Source: CAD feature listing. Evaluate the final solid. Frame: model axes, mm. A direction names the side the tool comes from. Give positions to 0.01 mm unless a question says otherwise; leave off trailing zeros. Loops run counter-clockwise (first coordinate to the right, second up) from the corner with the lowest first, then second, coordinate; pieces in that order, holes last.
from build123d import *

# Parameters (mm, degrees)
SKETCH1_W               = 120
SKETCH1_H               = 100
BOSS_EXTRUDE1_DEPTH     = 5
SKETCH2_R               = 2.5
CUT_EXTRUDE1_DEPTH      = 6
CUT_EXTRUDE3_DEPTH      = 10
BOSS_EXTRUDE3_DEPTH     = 29.25
SKETCH8_W               = 20
SKETCH8_H               = 5
BOSS_EXTRUDE4_DEPTH     = 34.25
BOSS_EXTRUDE5_DEPTH     = 5
SKETCH11_W              = 5
SKETCH11_H              = 73
CUT_EXTRUDE6_DEPTH      = 1
CUT_EXTRUDE6_DEPTH_BACK = 120.837603572
SKETCH12_R              = 1.5
CUT_EXTRUDE7_DEPTH      = 69
CUT_EXTRUDE7_DEPTH_BACK = 6
SKETCH13_W              = 71.438611392
SKETCH13_H              = 5
BOSS_EXTRUDE6_DEPTH     = 10
SKETCH14_R              = 1.5
CUT_EXTRUDE8_DEPTH      = 30.25
SKETCH15_W              = 5
SKETCH15_H              = 14.999673458
SKETCH15_H_2            = 15
BOSS_EXTRUDE7_DEPTH     = 10
SKETCH17_R              = 1.5
CUT_EXTRUDE9_DEPTH      = 30.25


with BuildPart() as part:
    # Sketch1 → Boss-Extrude1 (new body)
    with BuildSketch(Plane.XY):
        with Locations((60, 50)):
            Rectangle(SKETCH1_W, SKETCH1_H)
    extrude(amount=BOSS_EXTRUDE1_DEPTH)

    # Sketch2 → Cut-Extrude1 (cut, through all)
    with BuildSketch(Plane.XY.offset(5)):
        with Locations((48.561388608, 53.909722104)):
            Circle(SKETCH2_R)
        with BuildLine():
            ThreePointArc((83.119368898, 4.555811435), (92.903152754, 13.119153924), (100.621925378, 23.582127225))
            ThreePointArc((100.621925378, 23.582127225), (96.02283809, 41.016960064), (78.588005251, 36.417872775))
            ThreePointArc((78.588005251, 36.417872775), (74.136099049, 30.383211826), (68.493169771, 25.444188565))
            ThreePointArc((68.493169771, 25.444188565), (65.36208077, 7.686900437), (83.119368898, 4.555811435))
        make_face()
    extrude(amount=-CUT_EXTRUDE1_DEPTH, mode=Mode.SUBTRACT)

    # Sketch5 → Cut-Extrude3 (cut)
    with BuildSketch(Plane.XY.offset(5)):
        with BuildLine():
            Line((120, 73), (48.561388608, 73))
            ThreePointArc((48.561388608, 73), (36.862057433, 68.994958603), (30.071644393, 58.660308282))
            Line((30.071644393, 58.660308282), (15, 0))
            Line((15, 0), (0, 0))
            Line((0, 0), (0, 100))
            Line((0, 100), (120, 100))
            Line((120, 100), (120, 73))
        make_face()
    extrude(amount=-CUT_EXTRUDE3_DEPTH, mode=Mode.SUBTRACT)

    # Sketch7 → Boss-Extrude3 (add)
    with BuildSketch(Plane(origin=(0, 0, 0), x_dir=(-1, 0, 0), z_dir=(0, 0, -1))):
        Polygon((-15, 0), (-30.123935814, 58.863831587), (-34.614250087, 56.248022366), (-20.162396428, 0), align=None)
        with BuildLine():
            Line((-120, 73), (-48.561388608, 73))
            ThreePointArc((-48.561388608, 73), (-45.276527497, 72.715263777), (-42.089655421, 71.869548932))
            Line((-42.089655421, 71.869548932), (-44.799142753, 68))
            Line((-44.799142753, 68), (-120, 68))
            Line((-120, 68), (-120, 73))
        make_face()
    extrude(amount=BOSS_EXTRUDE3_DEPTH)

    # Sketch8 → Boss-Extrude4 (add, through all)
    with BuildSketch(Plane(origin=(0, 0, -29.25), x_dir=(-1, 0, 0), z_dir=(0, 0, -1))):
        with Locations((-10.162396428, 2.5)):
            Rectangle(SKETCH8_W, SKETCH8_H)
    extrude(amount=-BOSS_EXTRUDE4_DEPTH)

    # Sketch10 → Boss-Extrude5 (add)
    with BuildSketch(Plane(origin=(0, 0, 0), x_dir=(-1, 0, 0), z_dir=(0, 0, -1))):
        with BuildLine():
            Line((-45.069655622, 67.613667586), (-42.089655421, 71.869548932))
            ThreePointArc((-42.089655421, 71.869548932), (-34.697505551, 66.663289264), (-30.124971237, 58.863228407))
            Line((-30.124971237, 58.863228407), (-34.614250087, 56.248022366))
            ThreePointArc((-34.614250087, 56.248022366), (-38.409874026, 63.248233001), (-45.069655622, 67.613667586))
        make_face()
    extrude(amount=BOSS_EXTRUDE5_DEPTH)

    # Sketch11 → Cut-Extrude6 (cut, two sides)
    with BuildSketch(Plane(origin=(120, 0, 0), x_dir=(0, 0, -1), z_dir=(1, 0, 0))) as cut_extrude6_sk:
        with Locations((-2.5, 36.5)):
            Rectangle(SKETCH11_W, SKETCH11_H)
    extrude(amount=CUT_EXTRUDE6_DEPTH, mode=Mode.SUBTRACT)
    extrude(cut_extrude6_sk.sketch, amount=-CUT_EXTRUDE6_DEPTH_BACK, mode=Mode.SUBTRACT)

    # Sketch12 → Cut-Extrude7 (cut, two sides)
    with BuildSketch(Plane(origin=(0, 5, 0), x_dir=(1, 0, 0), z_dir=(0, 1, 0))) as cut_extrude7_sk:
        with Locations((7.662396428, 14.625)):
            Circle(SKETCH12_R)
    extrude(amount=CUT_EXTRUDE7_DEPTH, mode=Mode.SUBTRACT)
    extrude(cut_extrude7_sk.sketch, amount=-CUT_EXTRUDE7_DEPTH_BACK, mode=Mode.SUBTRACT)

    # Sketch13 → Boss-Extrude6 (add)
    with BuildSketch(Plane(origin=(0, 73, 0), x_dir=(1, 0, 0), z_dir=(0, 1, 0))):
        with Locations((84.280694304, 2.5)):
            Rectangle(SKETCH13_W, SKETCH13_H)
        with Locations((84.280694304, 26.75)):
            Rectangle(SKETCH13_W, SKETCH13_H)
    extrude(amount=BOSS_EXTRUDE6_DEPTH)

    # Sketch14 → Cut-Extrude8 (cut, through all)
    with BuildSketch(Plane.XY):
        with Locations((65, 78)):
            Circle(SKETCH14_R)
        with Locations((115, 78)):
            Circle(SKETCH14_R)
    extrude(amount=-CUT_EXTRUDE8_DEPTH, mode=Mode.SUBTRACT)

    # Sketch15 → Boss-Extrude7 (add)
    with BuildSketch(Plane(origin=(14.07111669, -3.615304337, 0), x_dir=(0, 0, 1), z_dir=(-0.968542434, 0.248848456, 0))):
        with Locations((-2.5, 57.008250348)):
            Rectangle(SKETCH15_W, SKETCH15_H)
        with Locations((-26.75, 57.008413619)):
            Rectangle(SKETCH15_W, SKETCH15_H_2)
    extrude(amount=BOSS_EXTRUDE7_DEPTH)

    # Sketch17 → Cut-Extrude9 (cut, through all)
    with BuildSketch(Plane.XY):
        with Locations((23.414860226, 52.844005614)):
            Circle(SKETCH17_R)
    extrude(amount=-CUT_EXTRUDE9_DEPTH, mode=Mode.SUBTRACT)


solid = part.part
1) Cut plane A-A (y = 78). Return loops of the section in (x, z), and give its area (3 significant figures).
Checks:
outline: (48.56, -29.25) - (63.5, -29.25) - (63.5, -24.25) - (48.56, -24.25) - close; (48.56, -5) - (63.5, -5) - (63.5, 0) - (48.56, 0) - close; (66.5, -29.25) - (113.5, -29.25) - (113.5, -24.25) - (66.5, -24.25) - close; (66.5, -5) - (113.5, -5) - (113.5, 0) - (66.5, 0) - close; (116.5, -29.25) - (120, -29.25) - (120, -24.25) - (116.5, -24.25) - close; (116.5, -5) - (120, -5) - (120, 0) - (116.5, 0) - close
area: 654 mm2
2) Reachability of faces 1 (the flat face through (23, 51, -5)), 2 (the flat face through (48.561, 78, -2)), 3 (the flat face through (25.35, 60.09, -2.53)), 4 (the flat face through (32.338, 57.574, -17.67)) from +Z, -Z, +X, -X, +Y, -Y: full face, straight path, thin tool, end or side. Return the list, or none.
Checks:
face 1: -X, +Y
face 2: +Z, -Z, -X, +Y
face 3: +Z, -Z, +Y
face 4: -Z, +X, +Y
3) Cut plane C-C (z = -25.5). Return loops of the section in (x, y), and give its area (3 significant figures).
Checks:
outline: (0.16, 0) - (20.16, 0) - (34.61, 56.25) - (30.12, 58.86) - (20.44, 61.35) - (16.71, 46.82) - (26.39, 44.34) - (16.28, 5) - (0.16, 5) - close; (42.09, 71.87) - (44.8, 68) - (120, 68) - (120, 83) - (48.56, 83) - (48.56, 73) arc R19.09 ccw to start; hole circle Ø3 at (23.41, 52.84); hole circle Ø3 at (65, 78); hole circle Ø3 at (115, 78)
area: 1,600 mm2
4) Contact query for flat-ended pins moving along their axis: P1, Ø8, axis at x = 98, y = 62, coming from the -Z side; P2, Ø1.5, axis at x = 100, z = -16, coming from the -Y side; P3, Ø4, axis at x = 65, y = 78, coming from the +Z side; P4, Ø2, axis at y = 9, z = -12.5, coming from the +X side. Output: stop coordinate, or through.
Checks:
P1: passes through
P2: stops at y = 68
P3: stops at z = 0
P4: stops at x = 22.73
5) Cut plane B-B (x = 65). Return loops of the section in (y, z), and give its area (3 significant figures).
Checks:
outline: (68, -29.25) - (76.5, -29.25) - (76.5, -24.25) - (73, -24.25) - (73, -5) - (76.5, -5) - (76.5, 0) - (68, 0) - close; (79.5, -29.25) - (83, -29.25) - (83, -24.25) - (79.5, -24.25) - close; (79.5, -5) - (83, -5) - (83, 0) - (79.5, 0) - close
area: 216 mm2
6) Cut plane D-D (x = 110.5). Return loops of the section in (y, z), and give its area (3 significant figures).
Checks:
outline: (68, -29.25) - (83, -29.25) - (83, -24.25) - (73, -24.25) - (73, -5) - (83, -5) - (83, 0) - (68, 0) - close
area: 246 mm2
7) Pull-direction query (X, two-part tool) for faces 5 (the flat face through (85, 73, -14)), 6 (the cylindrical face through (45.322, 72.723, -14.42)), 7 (the cylindrical face through (24.846, 53.295, -2.465)); classes: released by +X, released by -X, zero draft, split by the parting line, or undercut.
Checks:
face 5: zero draft
face 6: released by -X
face 7: undercut
8) Ray query, probe 1 along Z at (x, y) = (22, 56); probe 2 along Y at (x, z) = (115, -3.65); probe 3 along Y at (x, z) = (109, -14.5). Return the intervals inside material, ascending.
Checks:
probe 1: z = -29.25 to -24.25, -5 to 0
probe 2: y = 68 to 76.5, 79.5 to 83
probe 3: y = 68 to 73
